The model under review builds one solid part; all positions refer to its coordinate system, in mm. A direction names the side the tool comes from. Give positions to 0.01 mm unless a question says otherwise; leave off trailing zeros. Loops run counter-clockwise (first coordinate to the right, second up) from the corner with the lowest first, then second, coordinate; pieces in that order, holes last. Notation, with made-up numbers: M 27.25,76.25 L 69.25,76.25 A33 cw 69.25,104.25 Z; hole C 16.5,82 d1. An arc over 180 degrees is marked long. Put each result on its own line as item: value. Start each with the question number.
from build123d import *

# Parameters (mm, degrees)
SKETCH1_W           = 25.4
SKETCH1_H           = 12.7
BOSS_EXTRUDE1_DEPTH = 2.54
FILLET1_R           = 0.635
SHELL1_START        = 0.635
SHELL1_OUTLINE_W    = 1.905
SHELL1_OUTLINE_H    = 11.43
SHELL1_DEPTH        = 24.13
SKETCH2_R           = 2.54
BOSS_EXTRUDE2_DEPTH = 1.905


# Read off the part's stored shape, not the designer's step: Shell1
with BuildPart() as part:
    # Sketch1 → Boss-Extrude1 (new body)
    with BuildSketch(Plane(origin=(0, 0, 0), x_dir=(1, 0, 0), z_dir=(0, 1, 0))):
        with Locations((12.7, 6.35)):
            Rectangle(SKETCH1_W, SKETCH1_H)
    extrude(amount=BOSS_EXTRUDE1_DEPTH)

    # Fillet1
    fillet1_edges = [part.edges().sort_by_distance(p)[0] for p in [
        (0, 1.27, -12.7),
        (25.4, 1.27, -12.7),
        (25.4, 1.27, 0),
        (0, 1.27, 0),
    ]]
    fillet(fillet1_edges, radius=FILLET1_R)

    # Shell1 outline → Shell1 (cut)
    with BuildSketch(Plane.YZ.offset(SHELL1_START)):
        with Locations((0.9525, -6.35)):
            Rectangle(SHELL1_OUTLINE_W, SHELL1_OUTLINE_H)
    extrude(amount=SHELL1_DEPTH, mode=Mode.SUBTRACT)

    # Sketch2 → Boss-Extrude2 (add)
    with BuildSketch(Plane(origin=(0, 1.905, 0), x_dir=(-1, 0, 0), z_dir=(0, -1, 0))):
        with Locations(Location((-12.7, 6.35, 0), (0, 0, 270))):
            Circle(SKETCH2_R)
    extrude(amount=BOSS_EXTRUDE2_DEPTH)


solid = part.part
(1) We need section D-D, the plane z = -11.25. Write out the cut boundary in (x, y) (3 decimals).
(2) Insertion check: pin 1 (3.5 mm diameter, centred on x = 7, z = -4.5, fed in from -Y) (3 decimals). The pin has a flat end and moves straight along its axis. Give the tip position at first contact, or say it passes through.
(3) We need section B-B, the plane x = 12.7. Write out the cut boundary in (y, z) (3 decimals).
(4) Draft analysis for pull direction X (two halves, no side actions). For faces 3 (the flat face through (13, 0, -6)), 4 (the flat face through (13, 1, -0.635)), 5 (the flat face through (10, 1.905, -6)), 6 (the flat face through (25.4, 1, -6)), state which applies: +X half, -X half, draft (parallel to the pull), parting line (faces both ways), or undercut.
(5) For faces 1 (the flat face through (13, 1, 0)), 2 (the flat face through (0.635, 1, -6)), list the 3-axis set-ups (+Z, -Z, +X, -X, +Y, -Y) from which the entire face can be reached by the end or side of a thin tool; tool diameter is ignored.
(6) We need section C-C, the plane z = -6.35. Write out the cut boundary in (x, y) (3 decimals), plus the area to 3 significant figures.
(7) We need section A-A, the plane y = 1. Write out the cut boundary in (x, z) (3 decimals), plus the area to 3 significant figures.
(8) To check wall thickness, follow L1, parallel to X at y = 0.95, z = -8 (3 decimals); L2, parallel to X at y = 0.3, z = -2.75 (3 decimals); L3, parallel to Z at x = 18.25, y = 0.9 (3 decimals). State the ranges of each line that lie inside material, in increasing order. Write a range as [from, to].
Check sheet entries:
1. outline: M 0,0 L 0.635,0 L 0.635,1.905 L 24.765,1.905 L 24.765,0 L 25.4,0 L 25.4,2.54 L 0,2.54 Z
2. pin 1: stops at y = 1.905
3. outline: M 0,-12.7 L 2.54,-12.7 L 2.54,0 L 0,0 L 0,-0.635 L 1.905,-0.635 L 1.905,-3.81 L 0,-3.81 L 0,-8.89 L 1.905,-8.89 L 1.905,-12.065 L 0,-12.065 Z
4. face 3: draft
4. face 4: undercut
4. face 5: undercut
4. face 6: +X half
5. face 1: +Z, +X, -X, +Y, -Y
5. face 2: -Y
6. outline: M 0,0 L 0.635,0 L 0.635,1.905 L 10.16,1.905 L 10.16,0 L 15.24,0 L 15.24,1.905 L 24.765,1.905 L 24.765,0 L 25.4,0 L 25.4,2.54 L 0,2.54 Z
6. area: 28.2 mm²
7. outline: M 0,-12.065 A0.635 ccw 0.635,-12.7 L 24.765,-12.7 A0.635 ccw 25.4,-12.065 L 25.4,-0.635 A0.635 ccw 24.765,0 L 0.635,0 A0.635 ccw 0,-0.635 Z; C 12.7,-6.35 d5.08; hole M 0.635,-12.065 L 24.765,-12.065 L 24.765,-0.635 L 0.635,-0.635 Z
7. area: 66.7 mm²
8. L1: x = [0, 0.635], [10.769, 14.631], [24.765, 25.4]
8. L2: x = [0, 0.635], [24.765, 25.4]
8. L3: z = [-12.7, -12.065], [-0.635, 0]
